Build history of the part. All positions in model axes, mm. A direction names the side the tool comes from. Round coordinates to 2 decimals unless told otherwise and drop trailing zeros. Write each loop counter-clockwise with the first axis right and the second up, starting at its lowest first coordinate (ties: lowest second). Pieces come first, ordered by that corner, then holes.
1) Saw through at C-C (z = 1.95). Write the cut outline in (x, y).
2) Flat gauge pins, fed straight in: pin 1 (6 mm diameter, centred on x = 2.5, y = -5.5, fed in from +Z); pin 2 (10.5 mm diameter, centred on x = 0, y = 0, fed in from -Z); pin 3 (1.4 mm diameter, centred on x = -6, z = 2.5, fed in from +Y); pin 4 (1.4 mm diameter, centred on y = 0, z = 2.5, fed in from -X). Where does each tip first touch, or does it go through?
3) Which spindle directions (+Z, -Z, +X, -X, +Y, -Y) get a long thin tool onto all of the face, cutting with end or side? Do faces 1 (the flat face through (0, -10.561, 3)), 2 (the flat face through (27.3, 0, 3)), 3 (the flat face through (0, -10.141, 3)). Say none if no direction does.
4) Pull direction X, two halves, no side cores. Call faces 4 (the flat face through (-24.87, -8.08, 3.15)), 5 (the flat face through (0, 10.561, 3)), 6 (the flat face through (-27.3, 0, 3)): +X half, -X half, draft (parallel to the pull), parting line (faces both ways), or undercut.
5) Saw through at B-B (x = 0). Write the cut outline in (y, z).
6) Saw through at A-A (y = 0). Write the cut outline in (x, z).
7) Wall check: probe 1 along X at (y, z) = (-4, 2.4); probe 2 along Y at (x, z) = (0, 0.4); probe 3 along Y at (x, z) = (6, 3.3). Give the ranges that are in metal, low to high.
8) Saw through at D-D (x = 15.5). Write the cut outline in (y, z), plus the area to 3 significant figures.
from build123d import *

# Parameters (mm, degrees)
SKETCH1_W           = 56.769
SKETCH1_H           = 23.2918
BOSS_EXTRUDE1_DEPTH = 0.8
CUT_EXTRUDE1_DEPTH  = 1.8
BOSS_EXTRUDE2_DEPTH = 4.7625
SKETCH4_R           = 2.6162
CUT_EXTRUDE2_DEPTH  = 2.54
SKETCH5_R           = 4.1021
CUT_EXTRUDE3_DEPTH  = 2.54


with BuildPart() as part:
    # Sketch1 → Boss-Extrude1 (new body)
    with BuildSketch(Plane.XY):
        Rectangle(SKETCH1_W, SKETCH1_H)
    extrude(amount=BOSS_EXTRUDE1_DEPTH)

    # Sketch2 → Cut-Extrude1 (cut, through all)
    with BuildSketch(Plane.XY.offset(0.8)):
        Polygon((-28.3845, -6.696152532), (-23.434752532, -11.6459), (-28.3845, -11.6459), align=None)
        Polygon((-28.3845, 6.696152532), (-23.434752532, 11.6459), (-28.3845, 11.6459), align=None)
        Polygon((23.434752532, -11.6459), (28.3845, -6.696152532), (28.3845, -11.6459), align=None)
        Polygon((23.434752532, 11.6459), (28.3845, 6.696152532), (28.3845, 11.6459), align=None)
    extrude(amount=-CUT_EXTRUDE1_DEPTH, mode=Mode.SUBTRACT)

    # Sketch3 → Boss-Extrude2 (add)
    with BuildSketch(Plane.XY.offset(0.8)):
        Polygon((22.985413706, 10.561100114), (-22.985413706, 10.561100114), (-27.299700114, 6.246813706), (-27.299700114, -6.246813706), (-22.985413706, -10.561100114), (22.985413706, -10.561100114), (27.299700114, -6.246813706), (27.299700114, 6.246813706), align=None)
        Polygon((-22.81144401, 10.141100114), (-26.879700114, 6.07284401), (-26.879700114, -6.07284401), (-22.81144401, -10.141100114), (22.81144401, -10.141100114), (26.879700114, -6.07284401), (26.879700114, 6.07284401), (22.81144401, 10.141100114), align=None, mode=Mode.SUBTRACT)
    extrude(amount=BOSS_EXTRUDE2_DEPTH)

    # Sketch4 → Cut-Extrude2 (cut)
    with BuildSketch(Plane(origin=(0, 0, 0), x_dir=(-1, 0, 0), z_dir=(0, 0, -1))):
        with Locations((17.0307, 0)):
            Circle(SKETCH4_R)
    extrude(amount=-CUT_EXTRUDE2_DEPTH, mode=Mode.SUBTRACT)

    # Sketch5 → Cut-Extrude3 (cut)
    with BuildSketch(Plane(origin=(0, 0, 0), x_dir=(-1, 0, 0), z_dir=(0, 0, -1))):
        Circle(SKETCH5_R)
    extrude(amount=-CUT_EXTRUDE3_DEPTH, mode=Mode.SUBTRACT)


solid = part.part
Evaluation:
1. outline: (-27.3, -6.25) - (-22.99, -10.56) - (22.99, -10.56) - (27.3, -6.25) - (27.3, 6.25) - (22.99, 10.56) - (-22.99, 10.56) - (-27.3, 6.25) - close; hole (-26.88, -6.07) - (-22.81, -10.14) - (22.81, -10.14) - (26.88, -6.07) - (26.88, 6.07) - (22.81, 10.14) - (-22.81, 10.14) - (-26.88, 6.07) - close
2. pin 1: stops at z = 0.8
2. pin 2: stops at z = 0
2. pin 3: stops at y = 10.56
2. pin 4: stops at x = -27.3
3. face 1: +Z, +X, -X, -Y
3. face 2: +Z, +X, +Y, -Y
3. face 3: +Z
4. face 4: undercut
4. face 5: draft
4. face 6: -X half
5. outline: (-11.65, 0) - (-4.1, 0) - (-4.1, 0.8) - (-10.14, 0.8) - (-10.14, 5.56) - (-10.56, 5.56) - (-10.56, 0.8) - (-11.65, 0.8) - close; (4.1, 0) - (11.65, 0) - (11.65, 0.8) - (10.56, 0.8) - (10.56, 5.56) - (10.14, 5.56) - (10.14, 0.8) - (4.1, 0.8) - close
6. outline: (-28.38, 0) - (-19.65, 0) - (-19.65, 0.8) - (-26.88, 0.8) - (-26.88, 5.56) - (-27.3, 5.56) - (-27.3, 0.8) - (-28.38, 0.8) - close; (-14.41, 0) - (-4.1, 0) - (-4.1, 0.8) - (-14.41, 0.8) - close; (4.1, 0) - (28.38, 0) - (28.38, 0.8) - (27.3, 0.8) - (27.3, 5.56) - (26.88, 5.56) - (26.88, 0.8) - (4.1, 0.8) - close
7. probe 1: x = -27.3 to -26.88, 26.88 to 27.3
7. probe 2: y = -11.65 to -4.1, 4.1 to 11.65
7. probe 3: y = -10.56 to -10.14, 10.14 to 10.56
8. outline: (-11.65, 0) - (11.65, 0) - (11.65, 0.8) - (10.56, 0.8) - (10.56, 5.56) - (10.14, 5.56) - (10.14, 0.8) - (-10.14, 0.8) - (-10.14, 5.56) - (-10.56, 5.56) - (-10.56, 0.8) - (-11.65, 0.8) - close
8. area: 22.6 mm2
